```python
from build123d import *

# Parameters (mm, degrees)
BOSS_EXTRUDE1_DEPTH = 0.762


with BuildPart() as part:
    # Sketch1 → Boss-Extrude1 (new body)
    with BuildSketch(Plane.XY):
        with BuildLine():
            Line((-51.1725, -95.766078244), (-68, -95.766078244))
            Line((-68, -95.766078244), (-74.35, -89.416078244))
            Line((-74.35, -89.416078244), (-74.35, -60.234654728))
            Line((-74.35, -60.234654728), (-67.5, -60.234654728))
            ThreePointArc((-67.5, -60.234654728), (-63.19548747, -58.451667258), (-61.4125, -54.147154728))
            Line((-61.4125, -54.147154728), (-61.4125, -44.966078244))
            Line((-61.4125, -44.966078244), (-51.1725, -44.966078244))
            Line((-51.1725, -44.966078244), (-44.8225, -51.316078244))
            Line((-44.8225, -51.316078244), (-44.8225, -89.416078244))
            Line((-44.8225, -89.416078244), (-51.1725, -95.766078244))
        make_face()
    extrude(amount=BOSS_EXTRUDE1_DEPTH)


solid = part.part
```
Design review of the part built by this model. Coordinates are the model's own, in mm. Give positions to 0.01 mm unless a question says otherwise; leave off trailing zeros. Order: outer loops, then holes, each group sorted by start corner. A loop starts at its lowest first (then second) coordinate and runs counter-clockwise, first axis right, second up. Notation, with made-up numbers: (26, 20.5) -> (63, 20.5) arc R24 cw to (63, 53.5) -> close; hole circle Ø1 at (17.5, -2). An arc over 180 degrees is marked (long way). Write item = value, one per line. Start each with the question number.
(1) We need section B-B on x = -68.5. Write out the cut boundary in (y, z), plus the area to 3 significant figures.
(2) We need section C-C on y = -58.5. Write out the cut boundary in (x, z).
(3) To check wall thickness, follow line 1 along Y through (x, z) = (-68, 0.5); line 2 along Y through (x, z) = (-71.5, 0.7); line 3 along X through (y, z) = (-50.5, 0.35). State the ranges of each line that lie inside material, in increasing order.
Numbers:
q1.outline = (-95.27, 0) -> (-60.23, 0) -> (-60.23, 0.76) -> (-95.27, 0.76) -> close
q1.area = 26.7 mm^2
q2.outline = (-63.24, 0) -> (-44.82, 0) -> (-44.82, 0.76) -> (-63.24, 0.76) -> close
q3.line_1 = -95.77 to -60.23
q3.line_2 = -92.27 to -60.23
q3.line_3 = -61.41 to -45.64
